from build123d import *

# Parameters (mm, degrees)
F0_W     = 200
F0_H     = 86.747314
F0_R     = 10
F1_DEPTH = 15


with BuildPart() as f1:
    # F0 (on Front) → F1 (new body)
    with BuildSketch(Plane.XZ):
        with Locations((71.285965, -1.479412)):
            Rectangle(F0_W, F0_H)
        Circle(F0_R, mode=Mode.SUBTRACT)
        with Locations((100, 0)):
            Circle(F0_R, mode=Mode.SUBTRACT)
    extrude(amount=F1_DEPTH)


solid = f1.part
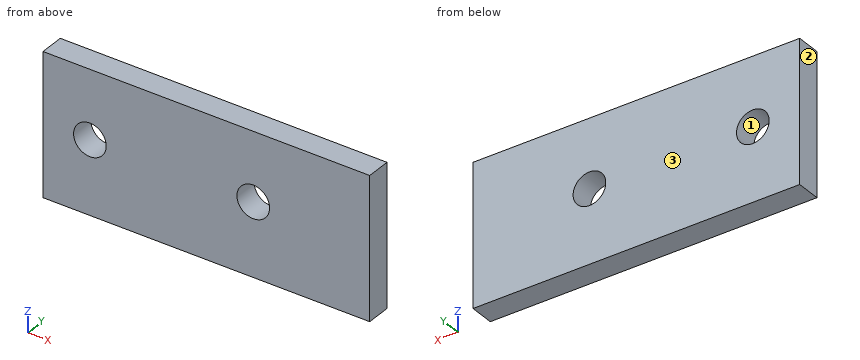
Build history of the part. All positions in model axes, mm. Face numbers are marked on the shaded views. Coordinates: 2 decimals unless noted, no trailing zeros. Order: outer loops, then holes, each group sorted by start corner. A loop starts at its lowest first (then second) coordinate and runs counter-clockwise, first axis right, second up. Notation, with made-up numbers: (1.5, 85) - (58.5, 85) arc R13 ccw to (58.5, 110) - close; hole circle Ø5 at (32, 3). An arc over 180 degrees is marked (long way). Write item = value, one per line. Start each with the question number.
1) Wall check: line 1 along Z through (x, y) = (100, -4.5); line 2 along X through (y, z) = (-12.75, 2); line 3 along Z through (x, y) = (96, -2). Give the ranges that are in metal, low to high. Write a range as from..to.
2) Saw through at A-A on z = 0. Write the cut outline in (x, y).
3) Saw through at B-B on x = 100. Write the cut outline in (y, z).
4) Two-plate mould, pull along X, no slides. Class the marked faces 1, 2 and 3: pulls with the +X half, pulls with the -X half, needs draft (parallel to the pull), parting line crosses it, or undercut.
5) Saw through at C-C on y = -2.5. Write the cut outline in (x, z), then the cut area to 3 significant figures.
From the geometry:
q1.line_1 = -44.85..-10, 10..41.89
q1.line_2 = -28.71..-9.8, 9.8..90.2, 109.8..171.29
q1.line_3 = -44.85..-9.17, 9.17..41.89
q2.outline = (-28.71, -15) - (-10, -15) - (-10, 0) - (-28.71, 0) - close; (10, -15) - (90, -15) - (90, 0) - (10, 0) - close; (110, -15) - (171.29, -15) - (171.29, 0) - (110, 0) - close
q3.outline = (-15, -44.85) - (0, -44.85) - (0, -10) - (-15, -10) - close; (-15, 10) - (0, 10) - (0, 41.89) - (-15, 41.89) - close
q4.face_1 = undercut
q4.face_2 = pulls with the -X half
q4.face_3 = needs draft
q5.outline = (-28.71, -44.85) - (171.29, -44.85) - (171.29, 41.89) - (-28.71, 41.89) - close; hole circle Ø20 at (0, 0); hole circle Ø20 at (100, 0)
q5.area = 16,700 mm^2
